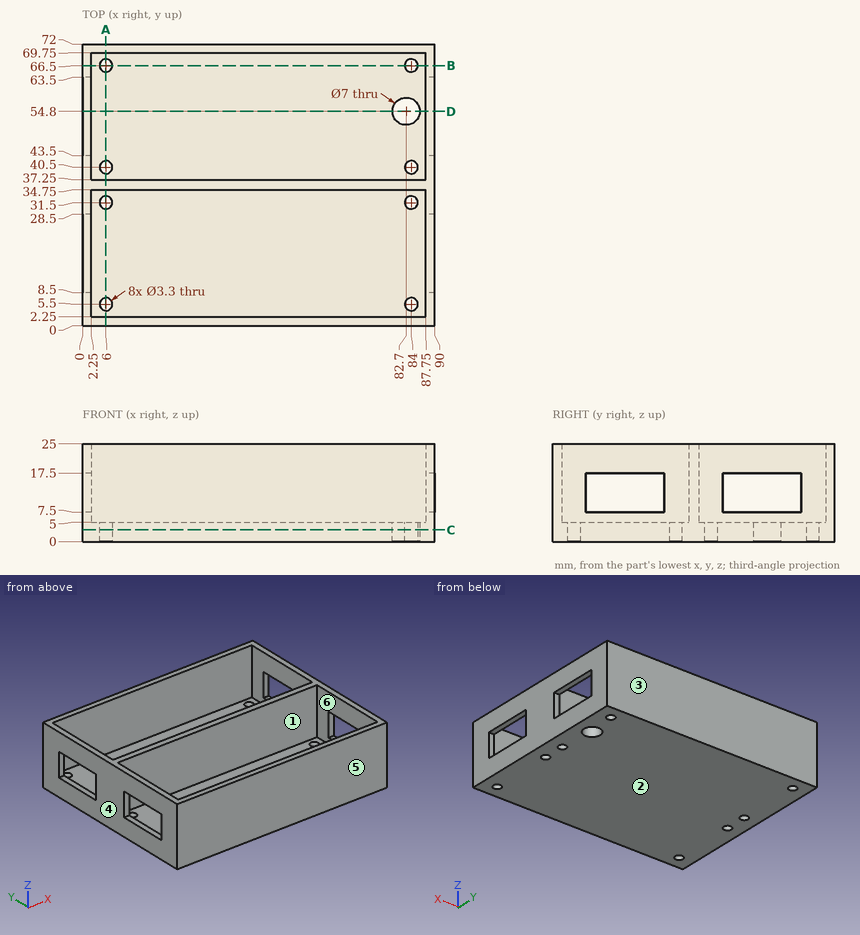
Print and shaded views of the part. All mm, measured from the part's lowest x, y and z. A direction names the side the tool comes from. Round coordinates to 2 decimals unless told otherwise and drop trailing zeros. Write each loop counter-clockwise with the first axis right and the second up, starting at its lowest first coordinate (ties: lowest second). Pieces come first, ordered by that corner, then holes.
Item 1: Cut at A-A, the plane x = 6. Give the cut face in (y, z), plus the area to 3 significant figures.
Results:
outline: (0, 0) - (3.85, 0) - (3.85, 5) - (2.25, 5) - (2.25, 25) - (0, 25) - close; (7.15, 0) - (29.85, 0) - (29.85, 5) - (7.15, 5) - close; (33.15, 0) - (38.85, 0) - (38.85, 5) - (37.25, 5) - (37.25, 25) - (34.75, 25) - (34.75, 5) - (33.15, 5) - close; (42.15, 0) - (64.85, 0) - (64.85, 5) - (42.15, 5) - close; (68.15, 0) - (72, 0) - (72, 25) - (69.75, 25) - (69.75, 5) - (68.15, 5) - close
area: 434 mm2
Item 2: Cut at C-C, the plane z = 3. Count the separate pieces of the cut face and the enclosed holes in it, plus the area to 3 significant figures.
Results:
separate pieces: 1
enclosed holes: 9
area: 6,370 mm2
Item 3: Cut at D-D, the plane y = 54.8. Give the cut face in (x, z).
Results:
outline: (0, 0) - (79.2, 0) - (79.2, 5) - (2.25, 5) - (2.25, 7.5) - (0, 7.5) - close; (0, 17.5) - (2.25, 17.5) - (2.25, 25) - (0, 25) - close; (86.2, 0) - (90, 0) - (90, 7.5) - (87.75, 7.5) - (87.75, 5) - (86.2, 5) - close; (87.75, 17.5) - (90, 17.5) - (90, 25) - (87.75, 25) - close
Item 4: Drop a flat-ended pin along its axis: pin 1 Ø4.5 at (x, y) = (6, 66.5) entering from +Z. Give the stop position or say it passes through.
Results:
pin 1: stops at z = 5
Item 5: Two-plate mould, pull along Y, no slides. Class the marked faces 3, 4, 5 and 6: +Y half, -Y half, draft (parallel to the pull), parting line (faces both ways), or undercut.
Results:
face 3: +Y half
face 4: draft
face 5: -Y half
face 6: undercut
Item 6: Which spindle directions (+Z, -Z, +X, -X, +Y, -Y) get a long thin tool onto all of the face, cutting with end or side? Do the marked faces 1 and 2. Say none if no direction does.
Results:
face 1: +Z
face 2: -Z, +X, -X, +Y, -Y
Item 7: Probe L1, parallel to Y at x = 4.5, z = 13.5; L2, parallel to X at y = 66.5, z = 3.55; L3, parallel to Y at x = 6, z = 3.9. List the from-to ranges inside material, lowest first.
Results:
L1: y = 0 to 2.25, 34.75 to 37.25, 69.75 to 72
L2: x = 0 to 4.35, 7.65 to 82.35, 85.65 to 90
L3: y = 0 to 3.85, 7.15 to 29.85, 33.15 to 38.85, 42.15 to 64.85, 68.15 to 72
Item 8: Cut at B-B, the plane y = 66.5. Give the cut face in (x, z), plus the area to 3 significant figures.
Results:
outline: (0, 0) - (4.35, 0) - (4.35, 5) - (2.25, 5) - (2.25, 25) - (0, 25) - close; (7.65, 0) - (82.35, 0) - (82.35, 5) - (7.65, 5) - close; (85.65, 0) - (90, 0) - (90, 25) - (87.75, 25) - (87.75, 5) - (85.65, 5) - close
area: 507 mm2
